Verification items for this drawing (mm, ordinates from the low corner). Coordinates: 2 decimals unless noted, no trailing zeros. Loops run counter-clockwise (first coordinate to the right, second up) from the corner with the lowest first, then second, coordinate; pieces in that order, holes last. Notation, with made-up numbers: (-18, 0) -> (-5, 0) arc R16 cw to (-5, 23) -> close; hole circle Ø2 at (-31, -37.75). An arc over 180 degrees is marked (long way). Write item = value, one per line.
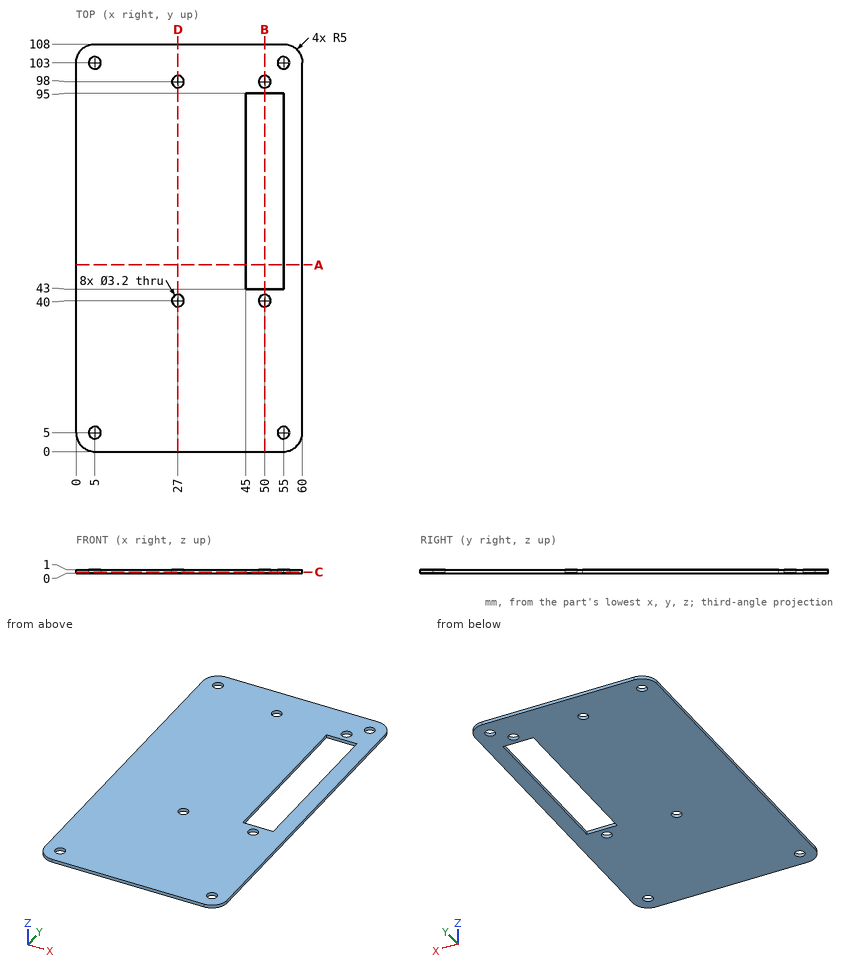
1) Sectioned sample at B-B, the plane x = 50. Record the cut outline in (y, z).
Ans:
outline = (0, 0) -> (38.4, 0) -> (38.4, 1) -> (0, 1) -> close; (41.6, 0) -> (43, 0) -> (43, 1) -> (41.6, 1) -> close; (95, 0) -> (96.4, 0) -> (96.4, 1) -> (95, 1) -> close; (99.6, 0) -> (108, 0) -> (108, 1) -> (99.6, 1) -> close
2) Sectioned sample at D-D, the plane x = 27. Record the cut outline in (y, z).
Ans:
outline = (0, 0) -> (38.4, 0) -> (38.4, 1) -> (0, 1) -> close; (41.6, 0) -> (96.4, 0) -> (96.4, 1) -> (41.6, 1) -> close; (99.6, 0) -> (108, 0) -> (108, 1) -> (99.6, 1) -> close
3) Sectioned sample at A-A, the plane y = 49.5. Record the cut outline in (x, z), plus the area to 3 significant figures.
Ans:
outline = (0, 0) -> (45, 0) -> (45, 1) -> (0, 1) -> close; (55, 0) -> (60, 0) -> (60, 1) -> (55, 1) -> close
area = 50.0 mm2
4) Sectioned sample at C-C, the plane z = 0.3. Count the separate pieces of the cut face and the enclosed holes in it, plus the area to 3 significant figures.
Ans:
separate_pieces = 1
enclosed_holes = 9
area = 5,870 mm2
5) Material ranges on line 1 (X direction, y = 103, z = 0.4); line 2 (Y direction, x = 27, z = 0.6); line 3 (X direction, y = 98, z = 0.3), recorded low to high.
Ans:
line_1 = 0 to 3.4, 6.6 to 53.4, 56.6 to 60
line_2 = 0 to 38.4, 41.6 to 96.4, 99.6 to 108
line_3 = 0 to 25.4, 28.6 to 48.4, 51.6 to 60
